Build history of the part. All positions in model axes, mm. Round coordinates to 2 decimals unless told otherwise and drop trailing zeros. Loops run counter-clockwise (first coordinate to the right, second up) from the corner with the lowest first, then second, coordinate; pieces in that order, holes last. Notation, with made-up numbers: (12, 23) - (36, 23) arc R17 cw to (36, 55) - close; hole circle Ø4 at (-39, 33.25). An arc over 180 degrees is marked (long way). Put each result on its own line as item: value. Start each with the question number.
from build123d import *

# Parameters (mm, degrees)
BOSS_EXTRUDE1_DEPTH = 1
BOSS_EXTRUDE2_DEPTH = 2
FILLET1_R           = 5


with BuildPart() as part:
    # Sketch1 → Boss-Extrude1 (new body)
    with BuildSketch(Plane(origin=(0, 0, 0), x_dir=(1, 0, 0), z_dir=(0, 1, 0))):
        with BuildLine():
            Line((-28.55625, 17.14897587), (28.55625, 17.14897587))
            ThreePointArc((28.55625, 17.14897587), (45.70522587, 0), (28.55625, -17.14897587))
            Line((28.55625, -17.14897587), (-28.55625, -17.14897587))
            ThreePointArc((-28.55625, -17.14897587), (-45.70522587, 0), (-28.55625, 17.14897587))
        make_face()
    extrude(amount=BOSS_EXTRUDE1_DEPTH)

    # Sketch2 → Boss-Extrude2 (add)
    with BuildSketch(Plane(origin=(0, 1, 0), x_dir=(1, 0, 0), z_dir=(0, 1, 0))):
        with BuildLine():
            Line((-28.55625, -7.14897587), (28.55625, -7.14897587))
            ThreePointArc((28.55625, -7.14897587), (35.70522587, 0), (28.55625, 7.14897587))
            Line((28.55625, 7.14897587), (-28.55625, 7.14897587))
            ThreePointArc((-28.55625, 7.14897587), (-35.70522587, 0), (-28.55625, -7.14897587))
        make_face()
    extrude(amount=BOSS_EXTRUDE2_DEPTH)

    # Fillet1
    # the kernel refuses this fillet: 5 mm, written as the material it takes off along each edge
    with BuildSketch(Plane(origin=(28.55625, 3, -7.14897587), x_dir=(0, -1, 0), z_dir=(-1, 0, 0)), Plane(origin=(-28.55625, 3, 7.14897587), x_dir=(0, -1, 0), z_dir=(1, 0, 0))) as fillet1_piece_1:
        with BuildLine():
            CenterArc((5, 4), FILLET1_R, 180, 53.130102354)
            Line((0, 4), (-0.1, 4))
            Line((-0.1, 4), (-0.1, 0))
            Line((-0.1, 0), (0, -0.1))
            ThreePointArc((0, -0.1), (1, -0.1), (1.94, -0.08))
            Line((1.94, -0.08), (2, 0))
        make_face()
    extrude(amount=57.1125, mode=Mode.SUBTRACT)
    with BuildSketch(Plane(origin=(28.55625, 3, 0), x_dir=(0, 0, 1), z_dir=(-1, 0, 0))) as fillet1_piece_2:
        with BuildLine():
            CenterArc((3.14897587, -5), FILLET1_R, 36.869897646, 53.130102354)
            Line((3.14897587, 0), (3.14897587, 0.1))
            Line((3.14897587, 0.1), (7.14897587, 0.1))
            Line((7.14897587, 0.1), (7.24897587, 0))
            ThreePointArc((7.24897587, 0), (7.24897587, -1), (7.22897587, -1.94))
            Line((7.22897587, -1.94), (7.14897587, -2))
        make_face()
    revolve(axis=Axis((28.55625, 3, 0), (0, 1, 0)), revolution_arc=180, mode=Mode.SUBTRACT)
    with BuildSketch(Plane(origin=(-28.55625, 3, 0), x_dir=(0, 0, -1), z_dir=(1, 0, 0))) as fillet1_piece_3:
        with BuildLine():
            CenterArc((3.14897587, -5), FILLET1_R, 36.869897646, 53.130102354)
            Line((3.14897587, 0), (3.14897587, 0.1))
            Line((3.14897587, 0.1), (7.14897587, 0.1))
            Line((7.14897587, 0.1), (7.24897587, 0))
            ThreePointArc((7.24897587, 0), (7.24897587, -1), (7.22897587, -1.94))
            Line((7.22897587, -1.94), (7.14897587, -2))
        make_face()
    revolve(axis=Axis((-28.55625, 3, 0), (0, 1, 0)), revolution_arc=180, mode=Mode.SUBTRACT)


solid = part.part
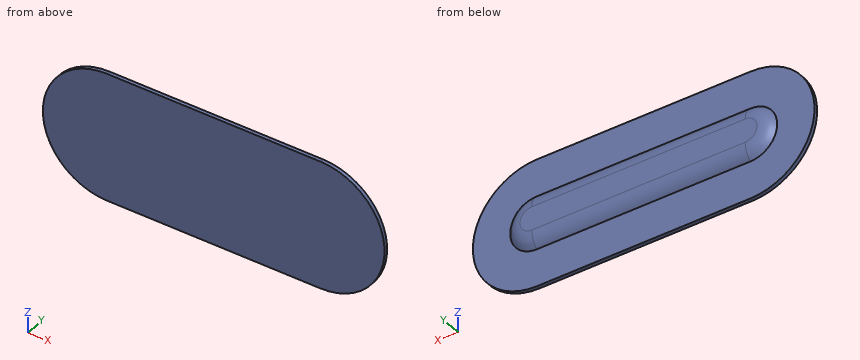
Item 1: Slice it at B-B (z = 12). Give the cut face in (x, y), plus the area to 3 significant figures.
Item 2: Drop flat-ended pins along their axis: pin 1 Ø1.5 at (x, y) = (-11, 2) entering from -Z; pin 2 Ø10 at (x, z) = (-9.5, -13) entering from +Y; pin 3 Ø4 at (x, z) = (5.5, -7.5) entering from +Y. Give the stop position or say it passes through.
Item 3: Slice it at A-A (x = 26.5). Give the cut face in (y, z), plus the area to 3 significant figures.
Item 4: Drill centre lines: probe 1 along Y at (x, z) = (-32, 7); probe 2 along Y at (x, z) = (-30, 3); probe 3 along Z at (x, y) = (-14, 1.05). Where is each one in solid material? Low to high. Write a range as [from, to].
Computed values:
1. outline: (-40.81, 0) - (40.81, 0) - (40.81, 1) - (-40.81, 1) - close
1. area: 81.6 mm^2
2. pin 1: stops at z = -6.95
2. pin 2: stops at y = 1
2. pin 3: stops at y = 2.41
3. outline: (0, -17.15) - (1, -17.15) - (1, -7.15) arc R5 ccw to (3, -3.15) - (3, 3.15) arc R5 ccw to (1, 7.15) - (1, 17.15) - (0, 17.15) - close
3. area: 58.1 mm^2
4. probe 1: y = [0, 1]
4. probe 2: y = [0, 3]
4. probe 3: z = [-7.11, 7.11]
